```python
from build123d import *

# Parameters (mm, degrees)
F0_W     = 38.1
F0_H     = 88.9
F1_DEPTH = 4.7625
F3_DEPTH = 12.7
F4_R     = 2.4003
F5_DEPTH = 9.525
F6_R     = 2.4003
F7_DEPTH = 9.525
F8_W     = 22.225
F8_H     = 48.26
F9_DEPTH = 9.526
F10_R    = 9.525


with BuildPart() as f1:
    # F0 (on Right) → F1 (new body, symmetric)
    with BuildSketch(Plane.YZ):
        with Locations((19.05, 44.45)):
            Rectangle(F0_W, F0_H)
    extrude(amount=F1_DEPTH, both=True)

    # F2 (on face) → F3 (cut, symmetric)
    with BuildSketch(Plane.YZ.offset(4.7625)):
        with BuildLine():
            Line((30.1625, 88.9), (7.9375, 88.9))
            Line((7.9375, 88.9), (7.9375, 76.835))
            ThreePointArc((7.9375, 76.835), (10.7273079092, 70.0998079092), (17.4625, 67.31))
            Line((17.4625, 67.31), (20.6375, 67.31))
            ThreePointArc((20.6375, 67.31), (27.3726920908, 70.0998079092), (30.1625, 76.835))
            Line((30.1625, 76.835), (30.1625, 88.9))
        make_face()
    extrude(amount=F3_DEPTH, both=True, mode=Mode.SUBTRACT)

    # F4 (on face) → F5 (cut)
    with BuildSketch(Plane.XY.offset(88.9)):
        with Locations((0, 3.96875)):
            Circle(F4_R)
        with Locations((0, 34.13125)):
            Circle(F4_R)
    extrude(amount=-F5_DEPTH, mode=Mode.SUBTRACT)

    # F6 (on face) → F7 (cut)
    with BuildSketch(Plane(origin=(0, 0, 0), x_dir=(1, 0, 0), z_dir=(0, 0, -1))):
        with Locations((0, -3.96875)):
            Circle(F6_R)
        with Locations((0, -34.13125)):
            Circle(F6_R)
    extrude(amount=-F7_DEPTH, mode=Mode.SUBTRACT)

    # F8 (on face) → F9 (cut, through all)
    with BuildSketch(Plane.YZ.offset(4.7625)):
        with Locations((19.05, 33.655)):
            Rectangle(F8_W, F8_H)
    extrude(amount=-F9_DEPTH, mode=Mode.SUBTRACT)

    # F10
    f10_edges = [f1.edges().sort_by_distance(p)[0] for p in [
        (0, 7.9375, 57.785),
        (0, 30.1625, 57.785),
        (0, 7.9375, 9.525),
        (0, 30.1625, 9.525),
    ]]
    fillet(f10_edges, radius=F10_R)


solid = f1.part
```
Here's how the part is built. I have some questions about the finished solid (model axes, mm). A direction names the side the tool comes from. Coordinates: 2 decimals unless noted, no trailing zeros. Loops run counter-clockwise (first coordinate to the right, second up) from the corner with the lowest first, then second, coordinate; pieces in that order, holes last. Notation, with made-up numbers: (-2, -30.5) - (38, -30.5) arc R28 cw to (38, -2.5) - close; hole circle Ø11 at (79, -2). An arc over 180 degrees is marked (long way). Return JSON: item names as keys, results as strings. Group by question number.
Item 1: We'd pull the mould along Y, two halves only. Please class faces 6 (the face through (4.762, 6, 45)), 7 (the face through (0, 19, 9.525)), 8 (the face through (0, 0, 44)): +Y half, -Y half, draft (parallel to the pull), parting line (faces both ways), or undercut.
Item 2: If we section it at C-C on y = 28: Write out the boundary of the cut face in (x, z).
Item 3: If we section it at A-A on z = 32.5: Write out the boundary of the cut face in (x, y).
Item 4: If we section it at D-D on z = 83: Write out the boundary of the cut face in (x, y).
Item 5: Will these pins go through, and if not, where does the flat tip stop? P1, Ø1.4, axis at x = -1, y = 4, coming from the +Z side (3 decimals); P2, Ø2.5, axis at x = 1.5, y = 19.5, coming from the +Z side; P3, Ø1.4, axis at x = 1, y = 33.5, coming from the -Z side (3 decimals).
Item 6: On a 3-axis mill with a long thin cutter (end or side, diameter ignored), from which of +Z, -Z, +X, -X, +Y, -Y can I reach the whole of each face in a straight line? I mean faces 1 (the face through (0, 7.938, 83)), 2 (the face through (-0.067, 27.298, 12.241)), 3 (the face through (-1.905, 5.429, 4.696)), 4 (the face through (0, 38.1, 44)), 5 (the face through (0, 4, 79.375)). Say none if no direction works.
Item 7: I need wall thicknesses on line 1 (Y direction, x = 0, z = 7); line 2 (Y direction, x = 0, z = 86.25); line 3 (Z direction, x = -1.5, y = 3.5) (3 decimals). Which ranges of each line are inside material? Lowest first, please. Write a range as from..to.
Calculated:
{
 "1": {"face 6": "draft", "face 7": "undercut", "face 8": "-Y half"},
 "2": {"outline": "(-4.76, 0) - (4.76, 0) - (4.76, 13.01) - (-4.76, 13.01) - close; (-4.76, 54.3) - (4.76, 54.3) - (4.76, 70.79) - (-4.76, 70.79) - close"},
 "3": {"outline": "(-4.76, 0) - (4.76, 0) - (4.76, 7.94) - (-4.76, 7.94) - close; (-4.76, 30.16) - (4.76, 30.16) - (4.76, 38.1) - (-4.76, 38.1) - close"},
 "4": {"outline": "(-4.76, 0) - (4.76, 0) - (4.76, 7.94) - (-4.76, 7.94) - close; (-4.76, 30.16) - (4.76, 30.16) - (4.76, 38.1) - (-4.76, 38.1) - close; hole circle Ø4.8 at (0, 3.97); hole circle Ø4.8 at (0, 34.13)"},
 "5": {"P1": "stops at z = 79.375", "P2": "stops at z = 67.31", "P3": "stops at z = 9.525"},
 "6": {"face 1": "+Z, +X, -X", "face 2": "+X, -X", "face 3": "-Z", "face 4": "+Z, -Z, +X, -X, +Y", "face 5": "+Z"},
 "7": {"line 1": "y = 0..1.57, 6.37..31.73, 36.53..38.1", "line 2": "y = 0..1.57, 6.37..7.94, 30.16..31.73, 36.53..38.1", "line 3": "z = 9.525..79.375"}
}
